```python
from build123d import *

# Parameters (mm, degrees)
SKETCH1_W           = 150
SKETCH1_H           = 132
SKETCH1_R           = 1.75
BOSS_EXTRUDE1_DEPTH = 5
SKETCH2_R           = 1.75
CUT_EXTRUDE1_DEPTH  = 5
SKETCH3_R           = 1.5
SKETCH3_R_2         = 1.64
SKETCH3_R_3         = 2.61
CUT_EXTRUDE2_DEPTH  = 5
SKETCH4_R           = 10.975
SKETCH4_R_2         = 13.275
CUT_EXTRUDE3_DEPTH  = 5


with BuildPart() as part:
    # Sketch1 → Boss-Extrude1 (new body)
    with BuildSketch(Plane(origin=(0, 0, 0), x_dir=(1, 0, 0), z_dir=(0, 1, 0))):
        Rectangle(SKETCH1_W, SKETCH1_H)
        with Locations(Location((71.997145932, 63.35748842, 0), (0, 0, 270))):
            Circle(SKETCH1_R, mode=Mode.SUBTRACT)
        with Locations(Location((71.997145932, -63.35748842, 0), (0, 0, 90))):
            Circle(SKETCH1_R, mode=Mode.SUBTRACT)
        with Locations(Location((-71.997145932, 63.35748842, 0), (0, 0, 90))):
            Circle(SKETCH1_R, mode=Mode.SUBTRACT)
        with Locations(Location((-71.997145932, -63.35748842, 0), (0, 0, 270))):
            Circle(SKETCH1_R, mode=Mode.SUBTRACT)
    extrude(amount=BOSS_EXTRUDE1_DEPTH)

    # Sketch2 → Cut-Extrude1 (cut)
    with BuildSketch(Plane.XZ):
        Polygon((-41.2, -26.8), (-41.2, 45.2), (-46.7, 45.2), (-46.7, 49.2), (-60.7, 49.2), (-60.7, 45.2), (-66.2, 45.2), (-66.2, -26.8), align=None)
        with Locations(Location((-39.3, 46.5, 0), (0, 0, 270))):
            Circle(SKETCH2_R)
        with Locations(Location((-39.3, -28.5, 0), (0, 0, 90))):
            Circle(SKETCH2_R)
        with Locations(Location((-69.8, 46.5, 0), (0, 0, 270))):
            Circle(SKETCH2_R)
        with Locations(Location((-69.8, -28.5, 0), (0, 0, 270))):
            Circle(SKETCH2_R)
    extrude(amount=-CUT_EXTRUDE1_DEPTH, mode=Mode.SUBTRACT)

    # Sketch3 → Cut-Extrude2 (cut)
    with BuildSketch(Plane(origin=(0, 5, 0), x_dir=(1, 0, 0), z_dir=(0, 1, 0))):
        with Locations(Location((-69.8, 51, 0), (0, 0, 270))):
            Circle(SKETCH3_R)
        with Locations(Location((-54.55, 51, 0), (0, 0, 270))):
            Circle(SKETCH3_R_2)
        with Locations(Location((-39.3, 51, 0), (0, 0, 270))):
            Circle(SKETCH3_R_3)
    extrude(amount=-CUT_EXTRUDE2_DEPTH, mode=Mode.SUBTRACT)

    # Sketch4 → Cut-Extrude3 (cut)
    with BuildSketch(Plane(origin=(0, 5, 0), x_dir=(1, 0, 0), z_dir=(0, 1, 0))):
        with Locations(Location((-11.7, 0, 0), (0, 0, 270))):
            Circle(SKETCH4_R)
        with Locations(Location((20.217797346, 43.3, 0), (0, 0, 270))):
            Circle(SKETCH4_R)
        with Locations(Location((20.217797346, -43.3, 0), (0, 0, 270))):
            Circle(SKETCH4_R)
        with Locations(Location((52.135594693, 0, 0), (0, 0, 270))):
            Circle(SKETCH4_R_2)
    extrude(amount=-CUT_EXTRUDE3_DEPTH, mode=Mode.SUBTRACT)


solid = part.part
```
Geometry check sheet. Reference: the model listing, model coordinates, mm. A direction names the side the tool comes from. Coordinates: 2 decimals unless noted, no trailing zeros. Write each loop counter-clockwise with the first axis right and the second up, starting at its lowest first coordinate (ties: lowest second). Pieces come first, ordered by that corner, then holes. Notation, with made-up numbers: M -27,42.25 L -22,42.25 A29 cw -22,78.25 Z; hole C 27.25,29.25 d7. An arc over 180 degrees is marked long. Use one line per item in the form item = value. Start each with the question number.
1) Set-up check for faces 1 (the flat face through (-54, 2, 49.2)), 2 (the flat face through (-75, 2, 1)): record each of +Z, -Z, +X, -X, +Y, -Y from which the full face is reachable in a straight line by a thin tool's end or side.
2) Release check for a two-part mould opening along Z. For faces 3 (the cylindrical face through (-55.55, 2.54, -52.3)), 4 (the flat face through (75, 2, 1)) record: pulls with the +Z half, pulls with the -Z half, needs draft (parallel to the pull), parting line crosses it, or undercut.
3) Section check B-B on x = -54.55. Enter the section's corners in (y, z).
4) Section check A-A on z = -28.5. Enter the section's corners in (x, y), and give its area (3 significant figures).
5) Thickness scan on probe 1 along X at (y, z) = (3.7, 0) (3 decimals); probe 2 along Z at (x, y) = (-69.8, 2.4); probe 3 along X at (y, z) = (2.45, -20.5). Record the ranges inside material, lowest first. Write a range as from..to.
6) Go/stop test with a flat-tipped pin: pin 1 Ø4.5 at (x, z) = (-69.8, -28.5) entering from -Y. Record where the tip stops, or that it passes through.
7) Section check C-C on z = 22. Enter the section's corners in (x, y).
8) Section check D-D on y = 1.7. State how many separate pieces and enclosed holes the cut face has, and give its area (3 significant figures).
Responses:
q1.face_1 = +Y, -Y
q1.face_2 = +Z, -Z, -X, +Y, -Y
q2.face_3 = undercut
q2.face_4 = needs draft
q3.outline = M 0,-66 L 5,-66 L 5,-52.64 L 0,-52.64 Z; M 0,-49.36 L 5,-49.36 L 5,-26.8 L 0,-26.8 Z; M 0,49.2 L 5,49.2 L 5,66 L 0,66 Z
q4.outline = M -75,0 L -71.55,0 L -71.55,5 L -75,5 Z; M -68.05,0 L -41.05,0 L -41.05,5 L -68.05,5 Z; M -37.55,0 L 75,0 L 75,5 L -37.55,5 Z
q4.area = 715 mm2
q5.probe_1 = -75..-66.2, -41.2..-22.675, -0.725..38.861, 65.411..75
q5.probe_2 = -66..-52.5, -49.5..-30.25, -26.75..44.75, 48.25..66
q5.probe_3 = -75..-66.2, -41.2..75
q6.pin_1 = 0
q7.outline = M -75,0 L -66.2,0 L -66.2,5 L -75,5 Z; M -41.2,0 L 75,0 L 75,5 L -41.2,5 Z
q8.separate_pieces = 1
q8.enclosed_holes = 16
q8.area = 16,100 mm2
